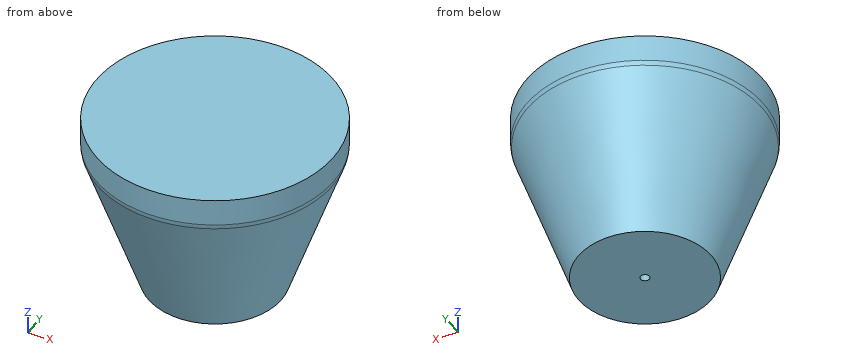
from build123d import *

# Parameters (mm, degrees)
F2_R     = 3
F3_DEPTH = 5
F4_R     = 10


with BuildPart() as f1:
    # F0 (on Front) → F1 (revolve)
    with BuildSketch(Plane.XZ):
        Polygon((0, 120), (0, 0), (45, 0), (80, 100), (80, 120), align=None)
    revolve(axis=Axis((0, 0, 170.90906), (0, 0, 1)))

    # F2 (on face) → F3 (cut)
    with BuildSketch(Plane(origin=(0, 0, 0), x_dir=(1, 0, 0), z_dir=(0, 0, -1))):
        Circle(F2_R)
    extrude(amount=-F3_DEPTH, mode=Mode.SUBTRACT)

    # F4
    f4_edges = [f1.edges().sort_by_distance(p)[0] for p in [
        (-80, 0, 100),
    ]]
    fillet(f4_edges, radius=F4_R)


solid = f1.part
Design review of the part built by this model. Coordinates are the model's own, in mm. Round coordinates to 2 decimals unless told otherwise and drop trailing zeros. Write each loop counter-clockwise with the first axis right and the second up, starting at its lowest first coordinate (ties: lowest second). Pieces come first, ordered by that corner, then holes.
Item 1: Consider section A-A on z = 72. Give the boundary of the cut face in (x, y), and give its area (3 significant figures).
Item 2: Wall thickness on L1, parallel to Y at x = 0, z = 2; L2, parallel to Y at x = 0, z = 1: over which ranges is each line inside the solid? List them lowest first.
Item 3: Consider section B-B on z = 111. Give the boundary of the cut face in (x, y), and give its area (3 significant figures).
Item 4: For pin 1 Ø5 at (x, y) = (1, -1) entering from -Z; pin 2 Ø5 at (x, z) = (-59, 60.5) entering from -Y; pin 3 Ø5 at (y, z) = (-22.5, 75.5) entering from +X; pin 4 Ø8 at (y, z) = (51, 90.5) entering from +X, all flat-tipped, find the tip position at first contact; note any pin that passes through.
Check values:
1. outline: circle Ø140.4 at (0, 0)
1. area: 15,500 mm2
2. L1: y = -45.7 to -3, 3 to 45.7
2. L2: y = -45.35 to -3, 3 to 45.35
3. outline: circle Ø160 at (0, 0)
3. area: 20,100 mm2
4. pin 1: stops at z = 0
4. pin 2: stops at y = -34.78
4. pin 3: stops at x = 69
4. pin 4: stops at x = 61.05
